For this review, take the finished solid that the model builds, in its own axes (mm). A direction names the side the tool comes from. Give positions to 0.01 mm unless a question says otherwise; leave off trailing zeros. Write each loop counter-clockwise with the first axis right and the second up, starting at its lowest first coordinate (ties: lowest second). Pieces come first, ordered by that corner, then holes. Notation, with made-up numbers: (-37.5, 40) -> (-1.5, 40) arc R28 ccw to (-1.5, 73) -> close; hole circle Ø5 at (-2.75, 8). An arc over 180 degrees is marked (long way). Write item = value, one per line.
Autodesk Inventor part; units mm, degrees
ref_plane "YZ Plane" through (0, 0, 0) normal (1, 0, 0) x (0, 1, 0)
ref_plane "XZ Plane" through (0, 0, 0) normal (0, 1, 0) x (-1, 0, 0)
ref_plane "XY Plane" through (0, 0, 0) normal (0, 0, 1) x (1, 0, 0)
sketch "Sketch1" plane through (0, 0, 0) normal (0, 1, 0) x (-1, 0, 0)
  line L0 (-17.5, 17.5) -> (17.5, 17.5)
  line L1 (17.5, 17.5) -> (17.5, -17.5)
  line L2 (17.5, -17.5) -> (-17.5, -17.5)
  line L3 (-17.5, -17.5) -> (-17.5, 17.5)
  line L4 (-17.5, 17.5) -> (17.5, -17.5) construction
  line L5 (17.5, 17.5) -> (-17.5, -17.5) construction
  circle A0 centre (12.5, -12.5) radius 1.65
  circle A1 centre (12.5, 12.5) radius 1.65
  circle A2 centre (-12.5, 12.5) radius 1.65
  circle A3 centre (-12.5, -12.5) radius 1.65
  circle A4 centre (0, 0) radius 6.05
  circle A5 centre (0, 0) radius 9.5
  circle A6 centre (0, 0) radius 12.7
  circle A7 centre (0, 0) radius 10.7
  dimension "d0" = 35
  dimension "d1" = 35
  dimension "d2" = 3.3
  dimension "d3" = 5
  dimension "d6" = 360
  dimension "d8" = 12.1
  dimension "d9" = 19
  dimension "d14" = 25.4
  dimension "d17" = 21.4
extrude "Extrusion1" add sketch "Sketch1" along normal blind 5 contours L0 L1 L2 L3 | A6
extrude "Extrusion2" add sketch "Sketch1" along normal blind 30 contours A5
extrude "Extrusion3" add sketch "Sketch1" along normal blind 17 contours A6 | A7
extrude "Extrusion4" cut sketch "Sketch1" along normal blind 10 contours A5 | A7
equation "\"d1\" = d0"
properties part number "test de tolerancia"
(1) Take a section at D-D (y = 28.25). Write out the cut boundary in (x, z).
Answers below:
outline = circle Ø19 at (0, 0); hole circle Ø12.1 at (0, 0)
(2) Take a section at A-A (z = 0). Write out the cut boundary in (x, y), plus the area to 3 significant figures.
Answers below:
outline = (-17.5, 0) -> (-10.7, 0) -> (-10.7, 10) -> (-6.05, 10) -> (-6.05, 30) -> (-9.5, 30) -> (-9.5, 17) -> (-12.7, 17) -> (-12.7, 5) -> (-17.5, 5) -> close; (6.05, 10) -> (10.7, 10) -> (10.7, 0) -> (17.5, 0) -> (17.5, 5) -> (12.7, 5) -> (12.7, 17) -> (9.5, 17) -> (9.5, 30) -> (6.05, 30) -> close
area = 271 mm^2
(3) Take a section at C-C (z = 11.5). Write out the cut boundary in (x, y).
Answers below:
outline = (-17.5, 0) -> (-13.81, 0) -> (-13.81, 5) -> (-17.5, 5) -> close; (-11.19, 0) -> (11.19, 0) -> (11.19, 5) -> (5.39, 5) -> (5.39, 17) -> (-5.39, 17) -> (-5.39, 5) -> (-11.19, 5) -> close; (13.81, 0) -> (17.5, 0) -> (17.5, 5) -> (13.81, 5) -> close
(4) The part is to be moulded in two halves that separate along Z. For faces 4 (the face through (-17.5, 2, 0)), 5 (the face through (2.75, 10.92, 12.4)), 6 (the face through (10.976, 2.465, 13.132)), say which applies: released by +Z, released by -Z, zero draft, split by the parting line, or undercut.
Answers below:
face_4 = zero draft
face_5 = split by the parting line
face_6 = undercut
(5) To check wall thickness, follow probe 1 along Y at (x, z) = (11.5, 4); probe 2 along X at (y, z) = (10.5, 0.5); probe 3 along Z at (x, y) = (0, 4). State the ranges of each line that lie inside material, in increasing order.
Answers below:
probe_1 = 0 to 17
probe_2 = -12.69 to -6.03, 6.03 to 12.69
probe_3 = -17.5 to -10.7, 10.7 to 17.5
(6) Take a section at B-B (x = -3.5). Write out the cut boundary in (y, z).
Answers below:
outline = (0, -17.5) -> (5, -17.5) -> (5, -12.21) -> (17, -12.21) -> (17, -8.83) -> (30, -8.83) -> (30, -4.93) -> (10, -4.93) -> (10, -10.11) -> (0, -10.11) -> close; (0, 10.11) -> (10, 10.11) -> (10, 4.93) -> (30, 4.93) -> (30, 8.83) -> (17, 8.83) -> (17, 12.21) -> (5, 12.21) -> (5, 17.5) -> (0, 17.5) -> close
(7) For pin 1 (3 mm diameter, centred on x = 12.5, z = 12.5, fed in from -Y); pin 2 (4 mm diameter, centred on x = -13.5, y = 15.5, fed in from -Z); pin 3 (5.5 mm diameter, centred on x = 12.5, z = -12.5, fed in from +Y); pin 4 (5 mm diameter, centred on x = 0.5, y = 16, fed in from +Z), all flat-tipped, find the tip position at first contact; note any pin that passes through.
Answers below:
pin_1 = through
pin_2 = -5.39
pin_3 = 5
pin_4 = 12.7
(8) Tool access review of faces 1 (the face through (8, 0, 8)), 2 (the face through (8, 5, 12)), 3 (the face through (2.32, 4.93, 10.446)): name each direction out of +Z, -Z, +X, -X, +Y, -Y from which nothing blocks a thin tool from reaching the whole face with its end or side.
Answers below:
face_1 = +Z, -Z, +X, -X, -Y
face_2 = +Y
face_3 = -Y
